For this review, take the finished solid that the model builds, in its own axes (mm). Face numbers are marked on the shaded views. A direction names the side the tool comes from. Coordinates: 2 decimals unless noted, no trailing zeros. Order: outer loops, then holes, each group sorted by start corner. A loop starts at its lowest first (then second) coordinate and runs counter-clockwise, first axis right, second up. Notation, with made-up numbers: (82, 42) -> (92, 42) arc R21 cw to (92, 56) -> close; hole circle Ø11 at (15, 87). An arc over 180 degrees is marked (long way). Return JSON: item names as keys, results as strings. Group by question number.
Item 1: Take a section at A-A (z = 1.55). Write out the cut boundary in (x, y), then the cut area to 3 significant figures.
Item 2: Take a section at C-C (y = 8). Write out the cut boundary in (x, z), then the cut area to 3 significant figures.
Item 3: For line 1 along Y through (x, z) = (5, 2.65); line 2 along X through (y, z) = (5, 1.35); line 3 along Z through (x, y) = (19.5, -3.5), list the stretches that pass through material, from the lowest coordinate up.
Item 4: Machinability: for the marked faces 1 and 2, which of the approach directions +Z, -Z, +X, -X, +Y, -Y give a long, thin tool a straight path to every point of the face, cutting with its end or side? Answer none if there is none.
Item 5: Insertion check: pin 1 (0.6 mm diameter, centred on y = 7, z = 1, fed in from +X); pin 2 (1.5 mm diameter, centred on y = -1.5, z = 3.5, fed in from -X); pin 3 (1.6 mm diameter, centred on x = 21, z = 3.5, fed in from -Y); pin 4 (3 mm diameter, centred on x = 5, y = 5, fed in from +Z). Each pin has a flat end and moves straight along its axis. Give the tip position at first contact, or say it passes through.
Item 6: Draft analysis for pull direction Y (two halves, no side actions). For the marked faces 3, 4 and 5, state which applies: +Y half, -Y half, draft (parallel to the pull), parting line (faces both ways), or undercut.
Item 7: Take a section at D-D (x = 13.25). Write out the cut boundary in (y, z).
Autodesk Fusion 360 part; units mm, degrees
sketch "Sketch1" plane through (0, 0, 0) normal (0, 0, 1) x (1, 0, 0)
  line L0 (0, 0) -> (8.5, 0)
  line L1 (8.5, 0) -> (8.5, 10)
  line L2 (8.5, 10) -> (0, 10)
  line L3 (0, 10) -> (0, 0)
  line L4 (0, 10) -> (10, 10)
  line L5 (10, 10) -> (10, 0)
  line L6 (10, 0) -> (0, 0)
  line L7 (0, 0) -> (0, 10)
  line L8 (0, 10) -> (10, 0)
  line L9 (0, 0) -> (10, 10)
  circle A0 centre (5, 5) radius 2
  dimension "d1" = 8.5
  dimension "d2" = 10
  dimension "d3" = 10
  dimension "d4" = 10
  dimension "d5" = 4
extrude "Extrude1" add sketch "Sketch1" along normal blind 2 contours L0 L1 L6 L8 L9 A0 | L3 L7 L8 L9 A0 | L1 L2 L4 L8 L9 A0 | L1 L8 L9 A0
sketch "Sketch2" plane through (0, 0, 2) normal (0, 0, 1) x (-1, 0, 0)
  circle A0 centre (-5, -5) radius 2
  line L0 (-8.5, 0) -> (-8.5, -10)
  line L1 (-8.5, -10) -> (0, -10)
  line L2 (0, -10) -> (0, 0)
  line L3 (0, 0) -> (-8.5, 0)
  line L4 (-8.5, -10) -> (-10, -10)
  line L5 (-10, -10) -> (-10, 0)
  line L6 (-10, 0) -> (-8.5, 0)
  line L7 (-8.5, 0) -> (-8.5, -10)
  line L8 (-10, -5) -> (-10, -18.25)
  line L9 (-10, -18.25) -> (-10, 8.25)
  line L10 (-10, -18.25) -> (-16.26, -18.25)
  line L11 (-16.26, -18.25) -> (-16.26, 8.25)
  line L12 (-16.26, 8.25) -> (-10, 8.25)
  line L13 (-10, 8.25) -> (-10, -18.25)
  line L14 (-16.26, 8.25) -> (-16.26, 4.75)
  line L15 (-16.26, 4.75) -> (-29.26, 4.75)
  line L16 (-29.26, 4.75) -> (-29.26, -14.25)
  line L17 (-29.26, -14.25) -> (-16.26, -14.25)
  line L18 (-16.26, -14.25) -> (-16.26, 4.75)
  dimension "d8" = 1.5
  dimension "d9" = 13.25
  dimension "d10" = 26.5
  dimension "d11" = 6.26
  dimension "d12" = 26.5
  dimension "d13" = 3.5
  dimension "d14" = 13
  dimension "d15" = 19
extrude "Extrude2" add sketch "Sketch2" along normal blind 2
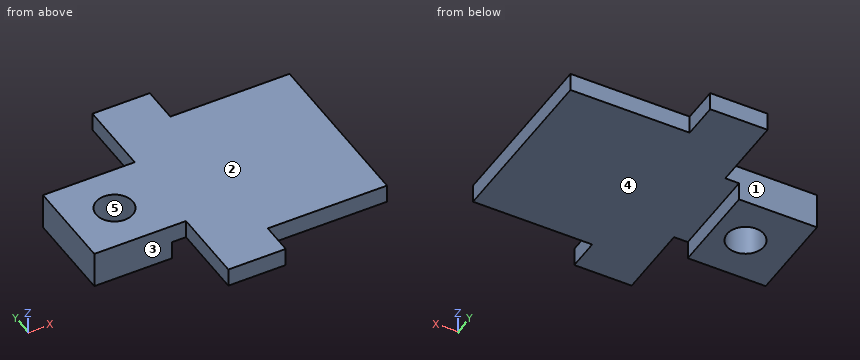
Findings below:
{
 "1": {"outline": "(0, 0) -> (8.5, 0) -> (8.5, 10) -> (0, 10) -> close; hole circle Ø4 at (5, 5)", "area": "72.4 mm2"},
 "2": {"outline": "(0, 0) -> (8.5, 0) -> (8.5, 2) -> (29.26, 2) -> (29.26, 4) -> (0, 4) -> close", "area": "75.5 mm2"},
 "3": {"line 1": "y = 0 to 3, 7 to 10", "line 2": "x = 0 to 3, 7 to 8.5", "line 3": "z = 2 to 4"},
 "4": {"face 1": "+Z, -Z, -X, +Y", "face 2": "+Z, +X, -X, +Y, -Y"},
 "5": {"pin 1": "stops at x = 8.5", "pin 2": "stops at x = 10", "pin 3": "stops at y = -4.75", "pin 4": "passes through"},
 "6": {"face 3": "-Y half", "face 4": "draft", "face 5": "undercut"},
 "7": {"outline": "(-8.25, 2) -> (18.25, 2) -> (18.25, 4) -> (-8.25, 4) -> close"}
}
